Geometry check sheet. Reference: the model listing, model coordinates, mm. A direction names the side the tool comes from. Coordinates: 2 decimals unless noted, no trailing zeros. Write each loop counter-clockwise with the first axis right and the second up, starting at its lowest first coordinate (ties: lowest second). Pieces come first, ordered by that corner, then holes. Notation, with made-up numbers: (81.5, -6.75) -> (101.5, -6.75) arc R17 ccw to (101.5, 6.25) -> close; hole circle Ø1 at (71, -31). An arc over 180 degrees is marked (long way). Use a Markdown table: item, result.
Autodesk Inventor part; units mm, degrees
ref_plane "YZ Plane" through (0, 0, 0) normal (1, 0, 0) x (0, 1, 0)
ref_plane "XZ Plane" through (0, 0, 0) normal (0, 1, 0) x (-1, 0, 0)
ref_plane "XY Plane" through (0, 0, 0) normal (0, 0, 1) x (1, 0, 0)
sketch "Sketch1" plane through (0, 0, 0) normal (0, 1, 0) x (-1, 0, 0)
  line L0 (2.286, 0) -> (10.414, 0)
  line L1 (12.7, -2.286) -> (12.7, -10.414)
  line L2 (10.414, -12.7) -> (2.286, -12.7)
  line L3 (0, -10.414) -> (0, -2.286)
  line L4 (8.1534, -4.0386) -> (4.5466, -4.0386)
  line L5 (4.0386, -4.5466) -> (4.0386, -8.1534)
  line L6 (4.5466, -8.6614) -> (8.1534, -8.6614)
  line L7 (8.6614, -8.1534) -> (8.6614, -4.5466)
  line L8 (10.414, 0) -> (12.7, -2.286)
  line L9 (12.7, -10.414) -> (10.414, -12.7)
  line L10 (2.286, -12.7) -> (0, -10.414)
  line L11 (2.286, 0) -> (0, -2.286)
  arc A0 (8.6614, -4.5466) -> (8.1534, -4.0386) centre (8.1534, -4.5466) ccw
  arc A1 (8.1534, -8.6614) -> (8.6614, -8.1534) centre (8.1534, -8.1534) ccw
  arc A2 (4.0386, -8.1534) -> (4.5466, -8.6614) centre (4.5466, -8.1534) ccw
  arc A3 (4.5466, -4.0386) -> (4.0386, -4.5466) centre (4.5466, -4.5466) ccw
  line L12 (8.1534, -4.5466) -> (4.5466, -8.1534) construction
  line L13 (12.7, -10.414) -> (0, -2.286) construction
  point P0 (0, 0)
  point P1 (12.7, -12.7)
  point P2 (12.7, 0)
  point P3 (0, -12.7)
  point P4 (4.0386, -8.6614)
  point P5 (8.6614, -8.6614)
  point P6 (6.35, -6.35)
  dimension "d1" = 12.7
  dimension "d2" = 4.6228
  dimension "d3" = 2.286
  dimension "d4" = 2.286
  dimension "d5" = 2.286
  dimension "d6" = 2.286
  dimension "d7" = 2.286
  dimension "d8" = 2.286
  dimension "d9" = 2.286
  dimension "d10" = 2.286
  dimension "d11" = 0.508
extrude "Body" add sketch "Sketch1" along normal blind 1.1906
sketch "Sketch2" plane through (0, 1.1906, 0) normal (0, 1, 0) x (1, 0, 0)
  arc A0 (-8.1534, 8.6614) -> (-8.6614, 8.1534) centre (-8.1534, 8.1534) ccw construction
  arc A1 (-4.5466, 4.0386) -> (-4.0386, 4.5466) centre (-4.5466, 4.5466) ccw construction
  circle A2 centre (-6.35, 6.35) radius 2.1844
  line L0 (-8.1534, 8.1534) -> (-4.5466, 4.5466) construction
  point P0 (0, 0)
  dimension "d14" = 4.3688
surface extrude "Circle" sketch "Sketch2" against normal up to surface (1.1906 mm away) shown yes curves A2
pattern_linear "Rectangular Pattern1" count 2 spacing 12.7 along (0, 0, -1) of "Body", "Circle"
equation "\"d22\" = d19"
Item 1: Section check D-D on z = -11.25. Record the boundary of the cut face in (x, y).
Answer block:
| item | result |
|---|---|
| outline | (-11.86, 0) -> (-0.84, 0) -> (-0.84, 1.19) -> (-11.86, 1.19) -> close |
Item 2: Section check B-B on x = -0.75. Record the boundary of the cut face in (y, z).
Answer block:
| item | result |
|---|---|
| outline | (0, -23.86) -> (1.19, -23.86) -> (1.19, -14.24) -> (0, -14.24) -> close; (0, -11.16) -> (1.19, -11.16) -> (1.19, -1.54) -> (0, -1.54) -> close |
Item 3: Section check A-A on z = -17.75. Record the boundary of the cut face in (x, y).
Answer block:
| item | result |
|---|---|
| outline | (-12.7, 0) -> (-8.66, 0) -> (-8.66, 1.19) -> (-12.7, 1.19) -> close; (-4.04, 0) -> (0, 0) -> (0, 1.19) -> (-4.04, 1.19) -> close |
Item 4: Tool access check on faces 1 (the flat face through (-12.7, 1, -19)), 2 (the flat face through (-1.159, 0.587, -24.273)), 3 (the flat face through (-11.573, 0.587, -11.541)), 4 (the flat face through (-1.159, 0.587, -13.827)), 5 (the flat face through (-6, 1, -21.361)). Record the directions out of +Z, -Z, +X, -X, +Y, -Y that give a thin tool (end or side, any length) a straight path to the whole face; none if there is none.
Answer block:
| item | result |
|---|---|
| face 1 | +Z, -Z, -X, +Y, -Y |
| face 2 | -Z, +X, +Y, -Y |
| face 3 | -X, +Y, -Y |
| face 4 | +X, +Y, -Y |
| face 5 | +Y, -Y |
Item 5: Thickness scan on L1, parallel to Z at x = -8, y = 0.55; L2, parallel to X at y = 0.15, z = -17.75; L3, parallel to Z at x = -1.75, y = 0.7. Record the ranges inside material, lowest first. Write a range as [from, to].
Answer block:
| item | result |
|---|---|
| L1 | z = [-25.4, -21.36], [-16.74, -8.66], [-4.04, 0] |
| L2 | x = [-12.7, -8.66], [-4.04, 0] |
| L3 | z = [-24.86, -13.24], [-12.16, -0.54] |
Item 6: Section check C-C on y = 0.2. Count the separate pieces of the cut face and the enclosed holes in it, then the cut area to 3 significant figures.
Answer block:
| item | result |
|---|---|
| separate pieces | 1 |
| enclosed holes | 2 |
| area | 259 mm^2 |
Item 7: Mould release check, pull along X, two halves, no side actions. Record for faces 6 (the flat face through (-11.541, 0.587, -1.127)), 7 (the flat face through (-1.159, 0.587, -11.573)), 8 (the flat face through (-8.661, 1, -6)): +X half, -X half, draft (parallel to the pull), parting line (faces both ways), or undercut.
Answer block:
| item | result |
|---|---|
| face 6 | -X half |
| face 7 | +X half |
| face 8 | undercut |
